Read the model definition and answer for the solid it produces. Units are mm, in the model's axes. A direction names the side the tool comes from. Give positions to 0.01 mm unless a question says otherwise; leave off trailing zeros. Order: outer loops, then holes, each group sorted by start corner. A loop starts at its lowest first (then second) coordinate and runs counter-clockwise, first axis right, second up. Notation, with made-up numbers: (-35, -30.5) - (-8, -30.5) arc R25 cw to (-8, -6.5) - close; hole circle Ø5 at (13.25, 52). An arc over 180 degrees is marked (long way). Use a Markdown table: item, result. Add a question column.
1. Consider L1, parallel to Y at x = 0, z = 0.7; L2, parallel to Z at x = -1.3, y = -0.65; L3, parallel to Z at x = 2.3, y = 0.3. Determine where each line is inside the solid, lowest interval first.
2. A cutting plane is placed at D-D on z = 1.95. Determine the outline of the cut face in (x, y), and give its area (3 significant figures).
3. A cutting plane is placed at C-C on z = 0.3. Determine the outline of the cut face in (x, y), and give its area (3 significant figures).
4. For a pull along X with two mould halves and no side action, classify faces 3 (the flat face through (1, -1, 1)), 4 (the flat face through (0, 0, 0.8)), 5 (the cylindrical face through (-0.75, 0.03, 2.63)) as released by +X, released by -X, zero draft, split by the parting line, or undercut.
5. A cutting plane is placed at A-A on x = 0. Determine the outline of the cut face in (y, z), and give its area (3 significant figures).
6. Flat-ended cylindrical pins translate along their axes: P1, Ø1.5, axis at x = 0, z = 3, coming from the -Y side; P2, Ø0.9, axis at x = 0, y = 0.5, coming from the -Z side; P3, Ø1.5, axis at x = 1.5, z = 1, coming from the -Y side. Find the tip coordinate at first contact, or state that the pin passes through.
7. Which of the six approach directions +Z, -Z, +X, -X, +Y, -Y give full straight-line access (tool end or side, diameter ignored) to faces 1 (the cylindrical face through (-3, 0.1, 0.5)), 2 (the cylindrical face through (-1.5, 0.07, 0.65))?
```python
from build123d import *

# Parameters (mm, degrees)
SKETCH_R     = 3
PAD_DEPTH    = 1
SKETCH001_R  = 0.75
PAD001_DEPTH = 3
SKETCH002_R  = 1.5
POCKET_DEPTH = 0.8
FILLET_R     = 0.2
FILLET001_R  = 0.5
CHAMFER_SIZE = 0.5


with BuildPart() as part:
    # Sketch → Pad (new body)
    with BuildSketch(Plane.XY):
        Circle(SKETCH_R)
    extrude(amount=PAD_DEPTH)

    # Sketch001 (on Face3 of Pad) → Pad001 (join)
    with BuildSketch(Plane.XY.offset(1)):
        Circle(SKETCH001_R)
    extrude(amount=PAD001_DEPTH)

    # Sketch002 → Pocket (cut)
    with BuildSketch(Plane.XY):
        Circle(SKETCH002_R)
    extrude(amount=POCKET_DEPTH, mode=Mode.SUBTRACT)

    # Fillet
    fillet_edges = [part.edges().sort_by_distance(p)[0] for p in [
        (-0.75, 0, 4),
    ]]
    fillet(fillet_edges, radius=FILLET_R)

    # Fillet001
    fillet001_edges = [part.edges().sort_by_distance(p)[0] for p in [
        (-0.75, 0, 1),
    ]]
    fillet(fillet001_edges, radius=FILLET001_R)

    # Chamfer
    chamfer_edges = [part.edges().sort_by_distance(p)[0] for p in [
        (-1.5, 0, 0),
    ]]
    chamfer(chamfer_edges, length=CHAMFER_SIZE)


solid = part.part
```
Output values:
| question | item | result |
|---|---|---|
| 1 | L1 | -3 to -1.5, 1.5 to 3 |
| 1 | L2 | 0.8 to 1 |
| 1 | L3 | 0 to 1 |
| 2 | outline | circle Ø1.5 at (0, 0) |
| 2 | area | 1.77 mm² |
| 3 | outline | circle Ø6 at (0, 0); hole circle Ø3.4 at (0, 0) |
| 3 | area | 19.2 mm² |
| 4 | face 3 | zero draft |
| 4 | face 4 | undercut |
| 4 | face 5 | split by the parting line |
| 5 | outline | (-3, 0) - (-2, 0) - (-1.5, 0.5) - (-1.5, 0.8) - (1.5, 0.8) - (1.5, 0.5) - (2, 0) - (3, 0) - (3, 1) - (1.25, 1) arc R0.5 cw to (0.75, 1.5) - (0.75, 3.8) arc R0.2 ccw to (0.55, 4) - (-0.55, 4) arc R0.2 ccw to (-0.75, 3.8) - (-0.75, 1.5) arc R0.5 cw to (-1.25, 1) - (-3, 1) - close |
| 5 | area | 7.94 mm² |
| 6 | P1 | y = -0.75 |
| 6 | P2 | z = 0.8 |
| 6 | P3 | y = -2.9 |
| 7 | face 1 | +Z, -Z |
| 7 | face 2 | -Z |
